from build123d import *

# Parameters (mm, degrees)
SKETCH_R        = 4
SKETCH_R_2      = 2.25
PAD_DEPTH       = 25
CHAMFER_SIZE    = 0.25
CHAMFER001_SIZE = 1.5


with BuildPart() as part:
    # Sketch → Pad (new body)
    with BuildSketch(Plane.XY):
        Circle(SKETCH_R)
        Circle(SKETCH_R_2, mode=Mode.SUBTRACT)
    extrude(amount=PAD_DEPTH)

    # Chamfer
    chamfer_edges = [part.edges().sort_by_distance(p)[0] for p in [
        (-4, 0, 0),
    ]]
    chamfer(chamfer_edges, length=CHAMFER_SIZE)

    # Chamfer001
    chamfer001_edges = [part.edges().sort_by_distance(p)[0] for p in [
        (-2.25, 0, 25),
    ]]
    chamfer(chamfer001_edges, length=CHAMFER001_SIZE)


solid = part.part
Can you work these out from the model? Positions are in its coordinate system, mm. Give positions to 0.01 mm unless a question says otherwise; leave off trailing zeros. Write each loop counter-clockwise with the first axis right and the second up, starting at its lowest first coordinate (ties: lowest second). Pieces come first, ordered by that corner, then holes. Notation, with made-up numbers: M 77.25,-16 L 90.25,-16 A27 cw 90.25,12 Z; hole C -40,-16.75 d6. An arc over 180 degrees is marked long. Answer in a Markdown table with one row per item. Add a question column.
Item 1: We'd pull the mould along Y, two halves only. Please class faces 1 (the flat face through (2, -2, 0)), 2 (the cylindrical face through (-0.29, 2.23, 11.59)), 3 (the cylindrical face through (-0.867, -3.905, 12.452)): released by +Y, released by -Y, zero draft, split by the parting line, or undercut.
Item 2: Please list where these lines run through material, in increasing order: L1, parallel to Y at x = 0, z = 18; L2, parallel to X at y = -1, z = 9.75; L3, parallel to Y at x = 0.75, z = 7.
Item 3: Imagine slicing it at A-A, the plane y = 0. Write out the boundary of the cut face in (x, z).
Item 4: Imagine slicing it at C-C, the plane z = 12. Write out the boundary of the cut face in (x, y).
Item 5: For pin 1 Ø4 at (x, z) = (-0.5, 20.5) entering from +Y, with a flat end and sliding along its axis, tell me the tip position at first contact or that it passes through.
Evaluation:
| question | item | result |
|---|---|---|
| 1 | face 1 | zero draft |
| 1 | face 2 | undercut |
| 1 | face 3 | split by the parting line |
| 2 | L1 | y = -4 to -2.25, 2.25 to 4 |
| 2 | L2 | x = -3.87 to -2.02, 2.02 to 3.87 |
| 2 | L3 | y = -3.93 to -2.12, 2.12 to 3.93 |
| 3 | outline | M -4,0.25 L -3.75,0 L -2.25,0 L -2.25,23.5 L -3.75,25 L -4,25 Z; M 2.25,0 L 3.75,0 L 4,0.25 L 4,25 L 3.75,25 L 2.25,23.5 Z |
| 4 | outline | C 0,0 d8; hole C 0,0 d4.5 |
| 5 | pin 1 | stops at y = 4 |
